Here's how the part is built. I have some questions about the finished solid (model axes, mm). Face numbers are marked on the shaded views. Round coordinates to 2 decimals unless told otherwise and drop trailing zeros. Order: outer loops, then holes, each group sorted by start corner. A loop starts at its lowest first (then second) coordinate and runs counter-clockwise, first axis right, second up. Notation, with made-up numbers: (70.5, 74) -> (127.5, 74) arc R15 ccw to (127.5, 102) -> close; hole circle Ø9 at (73.5, 10.5). An arc over 180 degrees is marked (long way). Answer in a Markdown table with one row per item.
```python
from build123d import *

# Parameters (mm, degrees)
F0_W      = 6.35
F0_H      = 146.05
F0_W_2    = 101.6
F0_H_2    = 6.35
F1_DEPTH  = 228.6
F4_DEPTH  = 101.6
F5_DEPTH  = 6.35
F7_W      = 69.85
F7_H      = 29.8027028753
F8_DEPTH  = 6.35
F6_W      = 69.85
F6_H      = 67.7882859973
F9_DEPTH  = 6.35
F10_DEPTH = 6.35
F12_DEPTH = 234.95
F13_R     = 3.175
F14_DEPTH = 6.35
F16_DEPTH = 20.32
F17_DEPTH = 6.35
F20_DEPTH = 6.35
F18_R     = 6
F21_DEPTH = 12.7
F23_DEPTH = 12.7


with BuildPart() as f1:
    # F0 (on Right) → F1 (new body)
    with BuildSketch(Plane.YZ):
        Polygon((-30.3053990938, 47.6320354104), (-30.3053990938, 41.2820354104), (14.1446009062, 41.2820354104), (14.1446009062, 47.6320354104), (7.7946009062, 47.6320354104), (7.7946009062, 193.6820354104), align=None)
        with Locations((10.9696009062, 120.6570354104)):
            Rectangle(F0_W, F0_H)
        with Locations((64.9446009062, 44.4570354104)):
            Rectangle(F0_W_2, F0_H_2)
    extrude(amount=F1_DEPTH)

    # F2 (on face) → F4 (join)
    with BuildSketch(Plane.YZ.offset(228.6)):
        Polygon((-128.6153139693, 73.2781001605), (-122.4709442896, 71.6752211137), (-120.8680652427, 77.8195907934), (-115.2579885786, 99.3248846724), (-109.6479119145, 120.8301785514), (-108.0450328676, 126.9745482311), (-114.1894025473, 128.577427278), align=None)
        Polygon((-122.4709442896, 71.6752211137), (-30.3053990938, 47.6320354104), (-28.7025200469, 53.7764050901), (-106.5976272263, 74.0968678326), (-120.8680652427, 77.8195907934), align=None)
    extrude(amount=-F4_DEPTH)

    # F3 (on face) → F5 (join)
    with BuildSketch(Plane.YZ.offset(228.6)):
        Polygon((-109.6479119145, 120.8301785514), (-69.2754185778, 110.2982237679), (-17.4823667187, 96.7869928482), (-15.8794876718, 102.9313625279), (-62.5744384004, 115.1126540223), (-83.4675541487, 120.5630320436), (-108.0450328676, 126.9745482311), align=None)
    extrude(amount=-F5_DEPTH)

    # F7 (on face) → F8 (cut, through all)
    with BuildSketch(Plane(origin=(0, -138.3183697556, 36.0830529797), x_dir=(1, 0, 0), z_dir=(0, -0.9676172724, 0.2524218971))):
        with Locations((174.625, 59.6911852871)):
            Rectangle(F7_W, F7_H)
    extrude(amount=-F8_DEPTH, mode=Mode.SUBTRACT)

    # F6 (on face) → F9 (cut, through all)
    with BuildSketch(Plane(origin=(0, 11.3059348332, 43.3394168605), x_dir=(1, 0, 0), z_dir=(0, 0.2524218971, 0.9676172724))):
        with Locations((174.625, -99.8529585577)):
            Rectangle(F6_W, F6_H)
    extrude(amount=-F9_DEPTH, mode=Mode.SUBTRACT)

    # F2 (on face) + F5_face (on face) + F0 (on Right) → F10 (join)
    with BuildSketch(Plane.YZ.offset(228.6)):
        Polygon((-83.4675541487, 120.5630320436), (-62.5744384004, 115.1126540223), (-30.6417442167, 127.6311188518), (-7.020366585, 136.8913266941), (-3.0564552968, 152.0863199656), align=None)
    with BuildSketch(Plane(origin=(228.6, -14.5704476362, 90.6728554843), x_dir=(0, 1, 0), z_dir=(1, 0, 0))):
        Polygon((22.3650485424, 103.0091799261), (-1.3090400356, 12.2585070436), (-99.6189549112, 37.9045717937), (-114.0448663331, -17.3947553238), (-15.7349514576, -43.0408200739), (-15.7349514576, -49.3908200739), (130.3150485424, -49.3908200739), (130.3150485424, -43.0408200739), (28.7150485424, -43.0408200739), (28.7150485424, 103.0091799261), align=None)
        Polygon((-2.9119190825, 6.1141373639), (-14.1320724107, -36.8964503942), (-106.2976176065, -12.8532646909), (-95.0774642783, 30.1573230671), align=None, mode=Mode.SUBTRACT)
    with BuildSketch(Plane.YZ):
        Polygon((-30.3053990938, 47.6320354104), (-30.3053990938, 41.2820354104), (14.1446009062, 41.2820354104), (14.1446009062, 47.6320354104), (7.7946009062, 47.6320354104), (7.7946009062, 193.6820354104), align=None)
        with Locations((64.9446009062, 44.4570354104)):
            Rectangle(F0_W_2, F0_H_2)
        with Locations((10.9696009062, 120.6570354104)):
            Rectangle(F0_W, F0_H)
    extrude(amount=-F10_DEPTH)

    # F11 (on face) → F12 (cut, through all)
    with BuildSketch(Plane(origin=(-6.35, 0, 0), x_dir=(0, -1, 0), z_dir=(-1, 0, 0))):
        Polygon((23.742887054, 47.6320354104), (18.5949307967, 67.3658677301), (-7.7946009062, 168.5257392579), (-7.7946009062, 73.7693533301), (-7.7946009062, 47.6320354104), align=None)
    extrude(amount=-F12_DEPTH, mode=Mode.SUBTRACT)

    # F13 (on face) → F14 (cut, through all)
    with BuildSketch(Plane(origin=(0, 0, 41.2820354104), x_dir=(1, 0, 0), z_dir=(0, 0, -1))):
        with BuildLine():
            ThreePointArc((110.906295836, 7.9551242506), (113.4283928169, 8.705126833), (114.518704164, 11.0998498276))
            ThreePointArc((114.518704164, 11.0998498276), (109.2590155112, 13.4945728222), (110.906295836, 7.9551242506))
        make_face()
        with Locations((110.906295836, -42.7196009062)):
            Circle(F13_R)
    extrude(amount=-F14_DEPTH, mode=Mode.SUBTRACT)

    # F15 (on face) → F16 (join)
    with BuildSketch(Plane(origin=(-6.35, 0, 0), x_dir=(0, -1, 0), z_dir=(-1, 0, 0))):
        Polygon((29.0230958563, 52.5475311542), (30.3053990938, 47.6320354104), (128.6153139693, 73.2781001605), (126.0507074943, 83.1090916481), (119.9063378146, 81.5062126012), (120.8680652427, 77.8195907934), (121.1886410521, 76.5907168574), align=None)
    extrude(amount=-F16_DEPTH)

    # F15 (on face) → F17 (join)
    with BuildSketch(Plane(origin=(-6.35, 0, 0), x_dir=(0, -1, 0), z_dir=(-1, 0, 0))):
        Polygon((27.7407926188, 57.463026898), (29.0230958563, 52.5475311542), (121.1886410521, 76.5907168574), (120.8680652427, 77.8195907934), (119.9063378146, 81.5062126012), (95.3288590957, 75.0946964137), (80.4160992001, 71.2044112235), align=None)
        Polygon((43.3673341555, 103.2638010329), (80.4160992001, 71.2044112235), (95.3288590957, 75.0946964137), (2.0947278686, 155.7729417735), (7.7533245088, 134.0816546527), align=None)
    extrude(amount=-F17_DEPTH)

    # F19 (on face) → F20 (cut)
    with BuildSketch(Plane(origin=(0, 14.1446009062, 0), x_dir=(-1, 0, 0), z_dir=(0, 1, 0))):
        Polygon((-73.025, 122.8082254529), (-73.025, 180.9820354104), (-114.1596585512, 180.9820354104), (-149.225, 180.9820354104), (-149.225, 126.8474459648), (-149.225, 60.3320354104), (-73.025, 60.3320354104), align=None)
    extrude(amount=-F20_DEPTH, mode=Mode.SUBTRACT)

    # F18 (on face) → F21 (cut)
    with BuildSketch(Plane(origin=(0, -40.0084548801, 10.4369882296), x_dir=(1, 0, 0), z_dir=(0, -0.9676172724, 0.2524218971))):
        with Locations((117.25, 68.4398338495)):
            Circle(F18_R)
        with Locations((105, 167.5570309162)):
            Circle(F18_R)
    extrude(amount=-F21_DEPTH, mode=Mode.SUBTRACT)

    # F22 (on face) → F23 (join)
    with BuildSketch(Plane(origin=(-6.35, 0, 0), x_dir=(0, -1, 0), z_dir=(-1, 0, 0))):
        Polygon((-14.1446009062, 171.4428658202), (-14.1446009062, 193.6820354104), (-115.7446009062, 47.6320354104), (-100.2738742348, 47.6320354104), (-84.3938715819, 70.4595392239), align=None)
    extrude(amount=-F23_DEPTH)


solid = f1.part
```
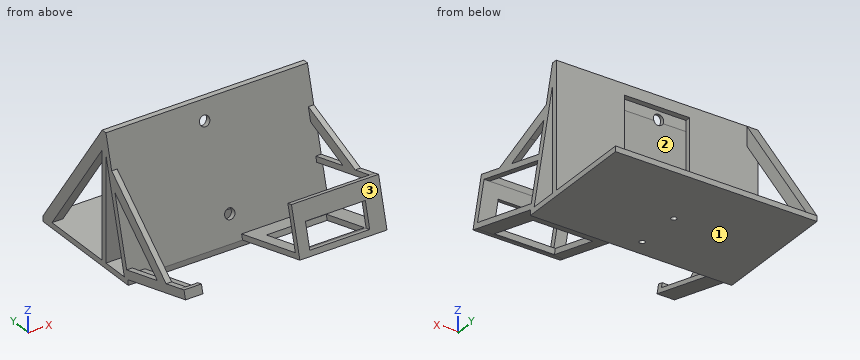
1. Please list where these lines run through material, in increasing order: line 1 along X through (y, z) = (-91.5, 69); line 2 along Y through (x, z) = (198, 124); line 3 along Z through (x, y) = (10, 84.5).
Numbers:
| item | result |
|---|---|
| line 1 | x = -6.35 to 0, 127 to 139.7, 209.55 to 228.6 |
| line 2 | y = -115.38 to -108.82, -10.38 to -3.82, 7.79 to 14.14 |
| line 3 | z = 41.28 to 47.63 |
2. Suppose I cut it at B-B on x = 60.5. Write out the boundary of the cut face in (y, z), then the cut area to 3 significant figures.
Numbers:
| item | result |
|---|---|
| outline | (-30.31, 41.28) -> (115.74, 41.28) -> (115.74, 47.63) -> (14.14, 47.63) -> (14.14, 193.68) -> (7.79, 193.68) -> (-30.31, 47.63) -> close; hole (-23.74, 47.63) -> (7.79, 47.63) -> (7.79, 168.53) -> close |
| area | 2,730 mm2 |
3. Suppose I cut it at A-A on x = 183.5. Write out the boundary of the cut face in (y, z), then the cut area to 3 significant figures.
Numbers:
| item | result |
|---|---|
| outline | (-128.62, 73.28) -> (-119.71, 70.96) -> (-118.11, 77.1) -> (-127.01, 79.42) -> close; (-119.49, 108.26) -> (-113.35, 106.66) -> (-108.05, 126.97) -> (-114.19, 128.58) -> close; (-54.12, 53.84) -> (-30.31, 47.63) -> (-30.31, 41.28) -> (115.74, 41.28) -> (115.74, 47.63) -> (14.14, 47.63) -> (14.14, 193.68) -> (7.79, 193.68) -> (-28.7, 53.78) -> (-52.52, 59.99) -> close; hole (-23.74, 47.63) -> (7.79, 47.63) -> (7.79, 168.53) -> close |
| area | 3,080 mm2 |
4. We'd pull the mould along Z, two halves only. Please class the marked faces 1, 2 and 3: released by +Z, released by -Z, zero draft, split by the parting line, or undercut.
Numbers:
| item | result |
|---|---|
| face 1 | released by -Z |
| face 2 | undercut |
| face 3 | released by +Z |
5. Suppose I cut it at D-D on y = -41. Write out the boundary of the cut face in (x, z), then the cut area to 3 significant figures.
Numbers:
| item | result |
|---|---|
| outline | (-6.35, 50.42) -> (13.97, 50.42) -> (13.97, 55.67) -> (0, 55.67) -> (0, 60.92) -> (-6.35, 60.92) -> close; (-6.35, 105.31) -> (0, 105.31) -> (0, 122.11) -> (-6.35, 122.11) -> close; (127, 50.42) -> (228.6, 50.42) -> (228.6, 56.98) -> (127, 56.98) -> close; (222.25, 102.92) -> (228.6, 102.92) -> (228.6, 109.48) -> (222.25, 109.48) -> close; (222.25, 123.57) -> (228.6, 123.57) -> (228.6, 137.21) -> (222.25, 137.21) -> close |
| area | 1,040 mm2 |
6. For pin 1 Ø3 at (x, z) = (123, 131) entering from -Y; pin 2 Ø1.9 at (x, z) = (77.5, 46) entering from -Y; pin 3 Ø6 at (x, z) = (86.5, 163.5) entering from -Y; pin 4 Ø12 at (y, z) = (-37.5, 60.5) entering from -X, each with a flat end and sliding along its axis, tell me the tip position at first contact or that it passes through.
Numbers:
| item | result |
|---|---|
| pin 1 | stops at y = -8.95 |
| pin 2 | stops at y = -30.31 |
| pin 3 | stops at y = -0.86 |
| pin 4 | stops at x = -6.35 |
7. Suppose I cut it at C-C on y = 51. Write out the boundary of the cut face in (x, z).
Numbers:
| item | result |
|---|---|
| outline | (-6.35, 41.28) -> (228.6, 41.28) -> (228.6, 47.63) -> (-6.35, 47.63) -> close; (-6.35, 118.46) -> (6.35, 118.46) -> (6.35, 140.7) -> (-6.35, 140.7) -> close |
